Solid Edge part; units mm, degrees
sketch "Sketch1" plane through (0, 0, 0) normal (0, 0, -1) x (-1, 0, 0)
  line L0 (-85.725, -85.725) -> (85.725, -85.725)
  line L1 (85.725, -85.725) -> (85.725, 85.725)
  line L2 (85.725, 85.725) -> (-85.725, 85.725)
  line L3 (-85.725, 85.725) -> (-85.725, -85.725)
extrude "ExtrudedProtrusion_18" add sketch "Sketch1" along normal blind 3
sketch "Sketch2" plane through (-85.725, 77.9118, -2) normal (-1, 0, 0) x (0, -1, 0)
  line L0 (-7.8132, 2) -> (163.6368, 2)
  line L1 (163.6368, 2) -> (163.6368, -2)
  line L2 (163.6368, -2) -> (-7.8132, -2)
  line L3 (-7.8132, -2) -> (-7.8132, 2)
extrude "Protrusion1" add sketch "Sketch2" along normal blind 15
sketch "Sketch3" plane through (85.725, -66.89, -2) normal (1, 0, 0) x (0, -1, 0)
  line L0 (-152.615, 1) -> (18.835, 1)
  line L1 (18.835, 1) -> (18.835, -3)
  line L2 (18.835, -3) -> (-152.615, -3)
  line L3 (-152.615, -3) -> (-152.615, 1)
extrude "Protrusion2" add sketch "Sketch3" along normal blind 15
sketch "Sketch4" plane through (0, 0, -3) normal (0, 0, -1) x (0, 1, 0)
  line L0 (85.725, 100.725) -> (65.725, 100.725)
  line L1 (65.725, 100.725) -> (65.725, 97.475)
  line L2 (65.725, 97.475) -> (85.725, 97.475)
  line L3 (85.725, 97.475) -> (85.725, 100.725)
  line L4 (85.725, -100.725) -> (65.725, -100.725)
  line L5 (65.725, -100.725) -> (65.725, -97.475)
  line L6 (65.725, -97.475) -> (85.725, -97.475)
  line L7 (85.725, -97.475) -> (85.725, -100.725)
extrude "Cutout1" cut sketch "Sketch4" against normal blind 20
sketch "Sketch5" plane through (100.725, -10, 6) normal (1, 0, 0) x (0, -1, 0)
  line L0 (75.725, 9) -> (55.725, 9)
  line L1 (55.725, 9) -> (55.725, 5)
  line L2 (55.725, 5) -> (75.725, 5)
  line L3 (75.725, 5) -> (75.725, 9)
extrude "ExtrudedProtrusion_23" add sketch "Sketch5" along normal mid plane 6
sketch "Sketch6" plane through (-100.725, -10, 6) normal (-1, 0, 0) x (0, 1, 0)
  line L0 (-75.725, 10) -> (-55.725, 10)
  line L1 (-55.725, 10) -> (-55.725, 6)
  line L2 (-55.725, 6) -> (-75.725, 6)
  line L3 (-75.725, 6) -> (-75.725, 10)
extrude "ExtrudedProtrusion_24" add sketch "Sketch6" along normal mid plane 6
sketch "Sketch7" plane through (0, 0, 0) normal (0, 0, 1) x (1, 0, 0)
  circle A0 centre (-86.8888, -69.9822) radius 1.5
  circle A1 centre (-22.6318, -69.9822) radius 1.5
  line L0 (-79.6818, 10.5074) -> (-29.1653, 10.5074)
  line L1 (-29.1653, 10.5074) -> (-29.1653, -71.5314)
  line L2 (-29.1653, -71.5314) -> (-79.6818, -71.5314)
  line L3 (-79.6818, -71.5314) -> (-79.6818, 10.5074)
  circle A2 centre (-6.7579, 25.6299) radius 1.3484
  circle A3 centre (88.5296, 25.6299) radius 1.5
  circle A4 centre (88.5296, -18.7118) radius 1.5
  circle A5 centre (-6.7579, -18.7118) radius 1.5
  circle A6 centre (-86.8888, 7.9402) radius 1.5
  circle A7 centre (-22.6318, 7.9402) radius 1.5
  line L4 (0, 56.9826) -> (82.443, 56.9826)
  line L5 (82.443, 56.9826) -> (82.443, -70.319)
  line L6 (82.443, -70.319) -> (0, -70.319)
  line L7 (0, -70.319) -> (0, 56.9826)
extrude "Cutout2" cut sketch "Sketch7" against normal blind 45
sketch "Sketch8" plane through (0, -85.725, -1.5) normal (0, -1, 0) x (1, 0, 0)
  line L0 (-74.682, -1.5) -> (-132.0067, -1.5)
  line L1 (-132.0067, -1.5) -> (-132.0067, -6.1664)
  line L2 (-132.0067, -6.1664) -> (-74.682, -6.1664)
  line L3 (-74.682, -6.1664) -> (-74.682, -1.5)
  line L4 (80.62, 1.5) -> (132.4635, 1.5)
  line L5 (132.4635, 1.5) -> (132.4635, 12.3328)
  line L6 (132.4635, 12.3328) -> (80.62, 12.3328)
  line L7 (80.62, 12.3328) -> (80.62, 1.5)
extrude "Cutout3" cut sketch "Sketch8" against normal blind 250
Verification items for the finished model (mm, model axes). Coordinates: 2 decimals unless noted, no trailing zeros. Loops run counter-clockwise (first coordinate to the right, second up) from the corner with the lowest first, then second, coordinate; pieces in that order, holes last. Notation, with made-up numbers: (58.25, 15) - (93.25, 15) arc R22 ccw to (93.25, 40) - close; hole circle Ø7 at (62.5, -29). An arc over 180 degrees is marked (long way). Answer as a JSON object with one key per item and string values.
(1) Cross-section at D-D, the plane z = -1.45. Count the separate pieces of the cut face and the enclosed holes in it, then the cut area to 3 significant figures.
Response:
{"separate pieces": "1", "enclosed holes": "10", "area": "19,800 mm²"}
(2) Cross-section at B-B, the plane y = 3.5. Record the boundary of the cut face in (x, z) (3 decimals).
Response:
{"outline": "(-100.725, -3) - (-79.682, -3) - (-79.682, 0) - (-100.725, 0) - close; (-29.165, -3) - (0, -3) - (0, 0) - (-29.165, 0) - close; (82.443, -3) - (100.725, -3) - (100.725, 0) - (82.443, 0) - close"}
(3) Scan lines: line 1 along X through (y, z) = (-27.5, -1.65) (3 decimals); line 2 along Y through (x, z) = (-53.5, -2.4) (3 decimals); line 3 along X through (y, z) = (35, -0.75) (3 decimals). Record each from-to range of solid material in increasing order.
Response:
{"line 1": "x = -100.725 to -79.682, -29.165 to 0, 82.443 to 100.725", "line 2": "y = -85.725 to -71.531, 10.507 to 85.725", "line 3": "x = -100.725 to 0, 82.443 to 100.725"}
(4) Cross-section at C-C, the plane y = 40.5. Record the boundary of the cut face in (x, z) (3 decimals), then the cut area to 3 significant figures.
Response:
{"outline": "(-100.725, -3) - (0, -3) - (0, 0) - (-100.725, 0) - close; (82.443, -3) - (100.725, -3) - (100.725, 0) - (82.443, 0) - close", "area": "357 mm²"}
(5) Cross-section at A-A, the plane x = 4. Record the boundary of the cut face in (y, z) (3 decimals).
Response:
{"outline": "(-85.725, -3) - (-70.319, -3) - (-70.319, 0) - (-85.725, 0) - close; (56.983, -3) - (85.725, -3) - (85.725, 0) - (56.983, 0) - close"}
(6) Go/stop test with flat-tipped pins: pin 1 Ø2.5 at (x, y) = (-86.89, -69.98) entering from +Z (3 decimals); pin 2 Ø4 at (x, y) = (88.53, -18.71) entering from +Z; pin 3 Ø1.5 at (x, z) = (98.5, -1) entering from +Y (3 decimals); pin 4 Ø1.5 at (y, z) = (32.5, -1.5) entering from +X (3 decimals). Record where each tip stops, or that it passes through.
Response:
{"pin 1": "passes through", "pin 2": "stops at z = 0", "pin 3": "stops at y = 65.725", "pin 4": "stops at x = 100.725"}
